Part print with two shaded views. Sizes in mm from the minimum x, y, z corner. A direction names the side the tool comes from. Round coordinates to 2 decimals unless told otherwise and drop trailing zeros. Order: outer loops, then holes, each group sorted by start corner. A loop starts at its lowest first (then second) coordinate and runs counter-clockwise, first axis right, second up. Notation, with made-up numbers: (-5, 1) - (21, 1) arc R19 cw to (21, 18) - close; hole circle Ø3 at (-36.5, 77). An arc over 180 degrees is marked (long way). Answer as CSV lines item,"result". Start each with the question number.
1. 3-axis set-ups, long thin cutter, end or side, ignore diameter. For the marked faces 1 and 2: which of +Z, -Z, +X, -X, +Y, -Y reach the whole face in a straight line?
2. Pin check, flat tips, straight feed: pin 1 Ø6 at (x, y) = (59.5, 38.5) entering from +Z (1 decimal); pin 2 Ø21 at (y, z) = (16, 24.5) entering from -X; pin 3 Ø3 at (x, y) = (88.5, 34.5) entering from +Z (1 decimal). Stop position of each tip, or through.
3. Band-saw the part on B-B on z = 50. List the corners of the cut face in (x, y), then the cut area to 3 significant figures.
4. Wall check: line 1 along Y through (x, z) = (72, 56); line 2 along Z through (x, y) = (42.5, 10.5) (1 decimal); line 3 along Z through (x, y) = (54.5, 23.5) (1 decimal). Give the ranges that are in metal, low to high. Write a range as [from, to].
5. Band-saw the part on C-C on x = 24.5. List the corners of the cut face in (y, z).
6. Band-saw the part on A-A on x = 44. List the corners of the cut face in (y, z).
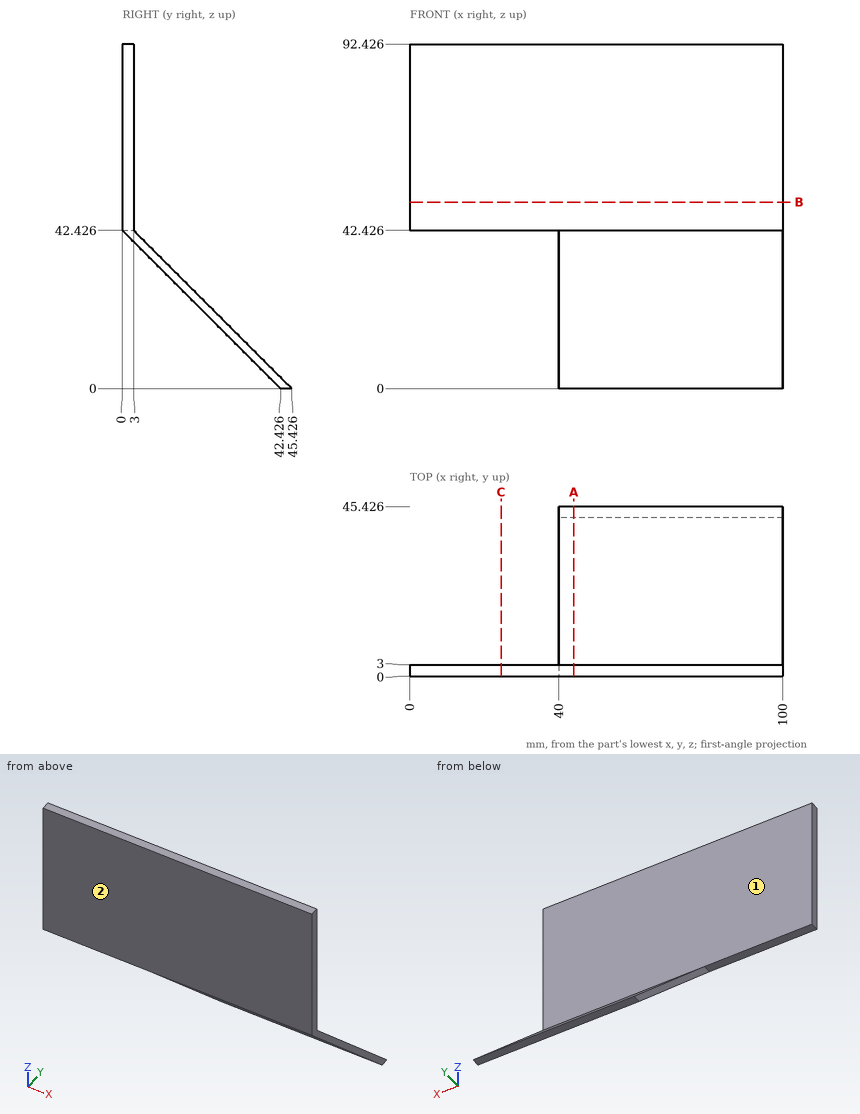
Reply:
1,face 1,"+Z, +X, -X, +Y"
1,face 2,"+Z, -Z, +X, -X, -Y"
2,pin 1,"stops at z = 9.9"
2,pin 2,"stops at x = 40"
2,pin 3,"stops at z = 12.4"
3,outline,"(0, 0) - (100, 0) - (100, 3) - (0, 3) - close"
3,area,"300 mm2"
4,line 1,"y = [0, 3]"
4,line 2,"z = [31.9, 34.9]"
4,line 3,"z = [18.9, 21.9]"
5,outline,"(0, 42.43) - (3, 42.43) - (3, 92.43) - (0, 92.43) - close"
6,outline,"(0, 42.43) - (42.43, 0) - (45.43, 0) - (3, 42.43) - (3, 92.43) - (0, 92.43) - close"
